Could you check a few things on this model? Use its own coordinates, in mm. Face numbers are marked on the shaded views. A direction names the side the tool comes from. Round coordinates to 2 decimals unless told otherwise and drop trailing zeros. Write each loop counter-clockwise with the first axis right and the second up, starting at its lowest first coordinate (ties: lowest second). Pieces come first, ordered by that corner, then holes. Notation, with made-up numbers: (54.25, -23) - (104.25, -23) arc R22 ccw to (104.25, 2) - close; hole circle Ø5 at (19.25, 9.5). An arc over 180 degrees is marked (long way). Write each question's results on one line, items separated by ' | '. Start each with the question number.
(1) Please list where these lines run through material, in increasing order: line 1 (X direction, y = -0.25, z = 3.75); line 2 (Y direction, x = -5.25, z = 7.5); line 3 (X direction, y = -2.25, z = 5.25). Write a range as [from, to].
(2) Imagine slicing it at B-B on x = 0. Write out the boundary of the cut face in (y, z), then the cut area to 3 significant figures.
(3) Imagine slicing it at A-A on y = 0. Write out the boundary of the cut face in (x, z).
(4) For P1, Ø2, axis at y = 3, z = 5.5, coming from the +X side; P2, Ø1, axis at x = 1, z = 6.5, coming from the +Y side; P3, Ø1.5, axis at y = -2, z = 6, coming from the -X side, each with a flat end and sliding along its axis, tell me the tip position at first contact or that it passes through.
(5) Imagine slicing it at C-C on z = 1.75. Write out the boundary of the cut face in (x, y).
(6) Imagine slicing it at D-D on y = 7.5. Write out the boundary of the cut face in (x, z), then the cut area to 3 significant figures.
(7) Thinking about a two-plate mould opening in Y: for the marked faces 3, 4 and 5, which applies, +Y half, -Y half, draft (parallel to the pull), parting line (faces both ways), or undercut?
(8) On a 3-axis mill with a long thin cutter (end or side, diameter ignored), from which of +Z, -Z, +X, -X, +Y, -Y can I reach the whole of each face in a straight line? I mean the marked faces 1 and 2. Say none if no direction works.
```python
from build123d import *

# Parameters (mm, degrees)
SKETCH_1_W            = 10
SKETCH_1_H            = 8
CUT_EXTRUDE_928_DEPTH = 6
CHAMFER_1_SIZE        = 1


with BuildPart() as part:
    # Sketch 1 → Revolve 1 (revolve)
    with BuildSketch(Plane(origin=(0, 0, 0), x_dir=(1, 0, 0), z_dir=(0, 1, 0)), mode=Mode.PRIVATE) as revolve_1_sk:
        with Locations((-5, -4)):
            Rectangle(SKETCH_1_W, SKETCH_1_H)
    revolve(revolve_1_sk.sketch.rotate(Axis((0, 0, 10.353242845), (0, 0, -1)), 180), axis=Axis((0, 0, 10.353242845), (0, 0, -1)))

    # Sketch 2 → Cut-Extrude 928 (cut)
    with BuildSketch(Plane(origin=(0, 0, 0), x_dir=(-1, 0, 0), z_dir=(0, 0, -1))):
        with BuildLine():
            Line((1.2489996, -1), (-1.2489996, -1))
            ThreePointArc((-1.2489996, -1), (0, 1.6), (1.2489996, -1))
        make_face()
    extrude(amount=-CUT_EXTRUDE_928_DEPTH, mode=Mode.SUBTRACT)

    # Chamfer 1
    chamfer_1_edges = [part.edges().sort_by_distance(p)[0] for p in [
        (0, 1.6, 0),
        (0, -1, 0),
    ]]
    chamfer(chamfer_1_edges, length=CHAMFER_1_SIZE)


solid = part.part
```
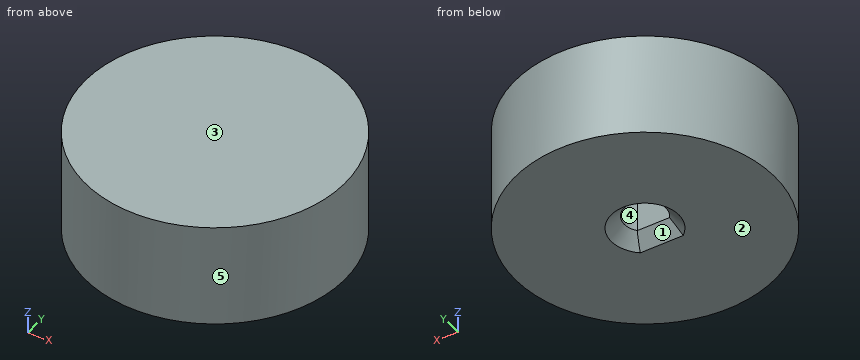
Response:
1) line 1: [-10, -1.58], [1.58, 10] | line 2: [-8.51, 8.51] | line 3: [-9.74, 9.74]
2) outline: (-10, 0) - (-2, 0) - (-1, 1) - (-1, 6) - (1.6, 6) - (1.6, 1) - (2.6, 0) - (10, 0) - (10, 8) - (-10, 8) - close | area: 143 mm²
3) outline: (-10, 0) - (-2.6, 0) - (-1.6, 1) - (-1.6, 6) - (1.6, 6) - (1.6, 1) - (2.6, 0) - (10, 0) - (10, 8) - (-10, 8) - close
4) P1: x = 9.8 | P2: y = 9.99 | P3: x = -9.92
5) outline: circle Ø20 at (0, 0); hole (-1.25, -1) - (1.25, -1) arc R1.6 ccw (long way) to start
6) outline: (-6.61, 0) - (6.61, 0) - (6.61, 8) - (-6.61, 8) - close | area: 106 mm²
7) face 3: draft | face 4: undercut | face 5: parting line
8) face 1: -Z | face 2: -Z, +X, -X, +Y, -Y
